```python
from build123d import *

# Parameters (mm, degrees)
BOSS_EXTRUDE1_DEPTH = 1.5875
SKETCH2_W           = 1.5875
SKETCH2_H           = 22.225
BOSS_EXTRUDE2_DEPTH = 6.5786
FILLET1_R           = 3.175
FILLET2_R           = 3.81
HOLE1_D             = 2.8448


with BuildPart() as part:
    # Sketch1 → Boss-Extrude1 (new body)
    with BuildSketch(Plane(origin=(0, 0, 0), x_dir=(1, 0, 0), z_dir=(0, 1, 0))):
        Polygon((8.9535, 28.575), (8.9535, 50.8), (10.541, 50.8), (10.541, 38.1), (40.259, 38.1), (40.259, 50.8), (41.8465, 50.8), (41.8465, 28.575), (50.8, 28.575), (50.8, 0), (0, 0), (0, 28.575), align=None)
    extrude(amount=BOSS_EXTRUDE1_DEPTH)

    # Sketch2 → Boss-Extrude2 (add)
    with BuildSketch(Plane(origin=(0, 1.5875, 0), x_dir=(1, 0, 0), z_dir=(0, 1, 0))):
        with Locations((9.74725, 39.6875)):
            Rectangle(SKETCH2_W, SKETCH2_H)
        with Locations((41.05275, 39.6875)):
            Rectangle(SKETCH2_W, SKETCH2_H)
    extrude(amount=BOSS_EXTRUDE2_DEPTH)

    # Fillet1
    fillet1_edges = [part.edges().sort_by_distance(p)[0] for p in [
        (9.74725, 0, -50.8),
        (41.05275, 0, -50.8),
        (9.74725, 8.1661, -50.8),
        (41.05275, 8.1661, -50.8),
    ]]
    fillet(fillet1_edges, radius=FILLET1_R)

    # Fillet2
    fillet2_edges = [part.edges().sort_by_distance(p)[0] for p in [
        (0, 0.79375, -28.575),
        (50.8, 0.79375, -28.575),
        (50.8, 0.79375, 0),
        (0, 0.79375, 0),
    ]]
    fillet(fillet2_edges, radius=FILLET2_R)

    # Hole1 (through all)
    with Locations(Plane.ZY.offset(-8.9535)):
        with Locations((-47.9552, 4.08305)):
            Hole(HOLE1_D / 2)


solid = part.part
```
CAD build for the part. Positions are in the model's coordinates, mm. A direction names the side the tool comes from. Coordinates: 2 decimals unless noted, no trailing zeros. Loops run counter-clockwise (first coordinate to the right, second up) from the corner with the lowest first, then second, coordinate; pieces in that order, holes last. Notation, with made-up numbers: (-6, -17.75) - (53, -17.75) arc R20 ccw to (53, -2.75) - close; hole circle Ø5 at (56.25, 72.5). An arc over 180 degrees is marked (long way). Return JSON: item names as keys, results as strings.
1. Band-saw the part on A-A (z = -30). Give the cut face in (x, y), and give its area (3 significant figures).
Result:
{"outline": "(8.95, 0) - (41.85, 0) - (41.85, 8.17) - (40.26, 8.17) - (40.26, 1.59) - (10.54, 1.59) - (10.54, 8.17) - (8.95, 8.17) - close", "area": "73.1 mm2"}
2. Band-saw the part on B-B (y = 6.75). Give the cut face in (x, z) (1 decimal), and give its area (3 significant figures).
Result:
{"outline": "(9, -50.3) - (10.5, -50.3) - (10.5, -28.6) - (9, -28.6) - close; (40.3, -50.3) - (41.8, -50.3) - (41.8, -28.6) - (40.3, -28.6) - close", "area": "68.9 mm2"}
3. Drop flat-ended pins along their axis: pin 1 (1.7 mm diameter, centred on y = 4.08, z = -47.96, fed in from -X); pin 2 (2 mm diameter, centred on y = 5.5, z = -28.5, fed in from +X); pin 3 (10 mm diameter, centred on x = 21.5, z = -27, fed in from +Y); pin 4 (1.3 mm diameter, centred on x = 26, y = 1, fed in from -Z). Give the stop position or say it passes through.
Result:
{"pin 1": "passes through", "pin 2": "stops at x = 41.85", "pin 3": "stops at y = 1.59", "pin 4": "stops at z = -38.1"}
4. 3-axis set-ups, long thin cutter, end or side, ignore diameter. For faces 1 (the flat face through (10, 5, -28.575)), 2 (the flat face through (40.259, 4, -40)), 3 (the flat face through (44, 1, -28.575)), 4 (the flat face through (6, 1, -28.575)), 5 (the cylindrical face through (9.758, 7.211, -49.895)): which of +Z, -Z, +X, -X, +Y, -Y reach the whole face in a straight line?
Result:
{"face 1": "+Z, +X, -X, +Y", "face 2": "-Z, +Y", "face 3": "-Z, +X, +Y, -Y", "face 4": "-Z, -X, +Y, -Y", "face 5": "-Z, +X, -X, +Y"}
5. Band-saw the part on D-D (z = -7). Give the cut face in (x, y), and give its area (3 significant figures).
Result:
{"outline": "(0, 0) - (50.8, 0) - (50.8, 1.59) - (0, 1.59) - close", "area": "80.6 mm2"}
6. Band-saw the part on C-C (x = 5.5). Give the cut face in (y, z) (1 decimal).
Result:
{"outline": "(0, -28.6) - (1.6, -28.6) - (1.6, 0) - (0, 0) - close"}
7. Mould opens along X. For faces 6 (the flat face through (41.846, 4, -40)), 7 (the flat face through (26, 1.588, -19)), 8 (the flat face through (26, 0, -19)) say: released by +X, released by -X, zero draft, split by the parting line, or undercut.
Result:
{"face 6": "released by +X", "face 7": "undercut", "face 8": "zero draft"}
8. Probe L1, parallel to X at y = 8, z = -34.5; L2, parallel to Y at x = 12.5, z = -19; L3, parallel to Z at x = 16, y = 0.5. List the from-to ranges inside material, lowest first. Write a range as from..to.
Result:
{"L1": "x = 8.95..10.54, 40.26..41.85", "L2": "y = 0..1.59", "L3": "z = -38.1..0"}
